Autodesk Inventor part; units mm, degrees
ref_plane "YZ Plane" through (0, 0, 0) normal (1, 0, 0) x (0, 1, 0)
ref_plane "XZ Plane" through (0, 0, 0) normal (0, 1, 0) x (-1, 0, 0)
ref_plane "XY Plane" through (0, 0, 0) normal (0, 0, 1) x (1, 0, 0)
sketch "Sketch1" plane through (0, 0, 0) normal (0, 0, 1) x (1, 0, 0)
  circle A0 centre (0, 0) radius 11.1125
  line L0 (0, 0) -> (7.6256, 0)
  line L1 (-3.8526, 6.604) -> (3.8128, 6.604)
  line L2 (3.8128, 6.604) -> (7.6256, 0)
  line L3 (7.6256, 0) -> (3.8128, -6.604)
  line L4 (3.8128, -6.604) -> (-3.8128, -6.604)
  line L5 (-3.8128, -6.604) -> (-7.6056, -0.0348)
  line L6 (-7.6056, -0.0348) -> (-3.8526, 6.604)
  line L7 (0, 0) -> (0, 6.604)
  line L8 (0, 0) -> (0, -6.604)
  line L9 (0, 0) -> (-5.7192, 3.302)
  line L10 (0, 0) -> (5.7192, -3.302)
  line L11 (0, 0) -> (5.7192, 3.302)
  line L12 (0, 0) -> (-5.7192, -3.302)
  line L13 (-7.2737, 0.1016) -> (-3.7248, 6.2484)
  line L14 (-3.5489, 6.35) -> (3.5489, 6.35)
  arc A1 (3.7248, 6.2484) -> (3.5489, 6.35) centre (3.5489, 6.1468) ccw
  line L15 (3.7248, 6.2484) -> (7.2737, 0.1016)
  arc A2 (-3.5489, 6.35) -> (-3.7248, 6.2484) centre (-3.5489, 6.1468) ccw
  arc A3 (-7.2737, 0.1016) -> (-7.2737, -0.1016) centre (-7.0977, 0) ccw
  line L16 (-3.7248, -6.2484) -> (-7.2737, -0.1016)
  line L17 (3.5489, -6.35) -> (-3.5489, -6.35)
  arc A4 (-3.7248, -6.2484) -> (-3.5489, -6.35) centre (-3.5489, -6.1468) ccw
  arc A5 (3.5489, -6.35) -> (3.7248, -6.2484) centre (3.5489, -6.1468) ccw
  line L18 (7.2737, -0.1016) -> (3.7248, -6.2484)
  arc A6 (7.2737, -0.1016) -> (7.2737, 0.1016) centre (7.0977, 0) ccw
  point P0 (0, 0)
  dimension "d0" = 22.225
  dimension "d19" = 6.604
  dimension "d20" = 6.604
  dimension "d21" = 6.604
  dimension "d22" = 6.604
  dimension "d23" = 60
  dimension "d24" = 60
  dimension "d25" = 6.604
  dimension "d26" = 6.604
  dimension "d27" = 60
  dimension "d28" = 60
  dimension "d30" = 13.208
extrude "Extrusion1" add sketch "Sketch1" along normal blind 12.7
sketch "Sketch3" plane through (-3.8128, -6.604, 0) normal (0, 1, 0) x (1, 0, 0)
  line L0 (11.4385, -12.7) -> (7.6256, -12.7)
  line L1 (7.6256, 0) -> (0, 0)
  line L2 (7.6256, -12.7) -> (0, 0)
  line L3 (7.6256, 0) -> (7.6256, -12.7)
  line L4 (0, 0) -> (7.6256, 0)
  line L5 (7.6256, 0) -> (7.6256, -12.7)
  line L6 (7.6256, -12.7) -> (0, -12.7)
  line L7 (7.6256, -12.7) -> (0, -12.7)
  line L8 (0, -12.7) -> (7.6256, 0)
  line L9 (0, 0) -> (0, -12.7)
  circle A0 centre (3.8128, -6.35) radius 1.27
  point P0 (3.8128, 0)
  dimension "d31" = 2.54
extrude "Extrusion2" cut sketch "Sketch3" against normal through all contours A0 L2 L8 | L8 L2 A0 | L2 L8 A0 | A0 L8 L2
properties part number "Churro Spacer"
Part model, mm, in its own coordinate system. A direction names the side the tool comes from. Coordinates: 2 decimals unless noted, no trailing zeros. Loops run counter-clockwise (first coordinate to the right, second up) from the corner with the lowest first, then second, coordinate; pieces in that order, holes last. Notation, with made-up numbers: M 26,33 L 36,33 A5 cw 36,37 Z; hole C 27.25,-29.5 d4. An arc over 180 degrees is marked long. Use a Markdown table: item, result. Add a question column.
Q1. Mould opens along Y. For faces 4 (the flat face through (0, -6.604, 8)), 5 (the cylindrical face through (10.6, -3.34, 6.26)), 6 (the flat face through (-5, -5, 12.7)) say: +Y half, -Y half, draft (parallel to the pull), parting line (faces both ways), or undercut.
Q2. Pin check, flat tips, straight feed: P1, Ø3, axis at y = 5.5, z = 5.5, coming from the -X side; P2, Ø4, axis at x = 2, z = 9, coming from the -Y side; P3, Ø6, axis at x = -3.5, z = 5.5, coming from the +Y side; P4, Ø3, axis at x = 5.5, z = 6.5, coming from the +Y side. Stop position of each tip, or through.
Q3. Cut at B-B (x = 6.25). Write the cut outline in (y, z), and give its area (3 significant figures).
Q4. Cut at D-D (x = 0). Write the cut outline in (y, z), and give its area (3 significant figures).
Q5. Probe L1, parallel to Z at x = 0, y = -10; L2, parallel to X at y = -1.75, z = 4; L3, parallel to X at y = -9.55, z = 6.35. List the from-to ranges inside material, lowest first.
Q6. Which spindle directions (+Z, -Z, +X, -X, +Y, -Y) get a long thin tool onto all of the face, cutting with end or side? Do faces 1 (the cylindrical face through (-0.28, -8.83, 7.59)), 2 (the flat face through (-5, -5, 0)), 3 (the flat face through (5.746, -3.256, 6.261)). Say none if no direction does.
Q7. Cut at A-A (y = 4.75). Write the cut outline in (x, z), and give its area (3 significant figures).
Q8. Cut at C-C (z = 2.5). Write the cut outline in (x, y) (1 decimal), and give its area (3 significant figures).
Worked out:
| question | item | result |
|---|---|---|
| 1 | face 4 | undercut |
| 1 | face 5 | parting line |
| 1 | face 6 | draft |
| 2 | P1 | stops at x = -10.37 |
| 2 | P2 | stops at y = -11.11 |
| 2 | P3 | stops at y = 11.1 |
| 2 | P4 | stops at y = 10.37 |
| 3 | outline | M -9.19,0 L -2.38,0 L -2.38,12.7 L -9.19,12.7 Z; M 2.38,0 L 9.19,0 L 9.19,12.7 L 2.38,12.7 Z |
| 3 | area | 173 mm2 |
| 4 | outline | M -11.11,0 L -6.6,0 L -6.6,5.08 L -11.11,5.08 Z; M -11.11,7.62 L -6.6,7.62 L -6.6,12.7 L -11.11,12.7 Z; M 6.6,0 L 11.11,0 L 11.11,12.7 L 6.6,12.7 Z |
| 4 | area | 103 mm2 |
| 5 | L1 | z = 0 to 5.08, 7.62 to 12.7 |
| 5 | L2 | x = -10.97 to -6.62, 6.62 to 10.97 |
| 5 | L3 | x = -5.68 to -1.27, 1.27 to 5.68 |
| 6 | face 1 | -Y |
| 6 | face 2 | -Z, +X, -X, +Y, -Y |
| 6 | face 3 | +Z, -Z |
| 7 | outline | M -10.05,0 L -4.9,0 L -4.9,12.7 L -10.05,12.7 Z; M 4.88,0 L 10.05,0 L 10.05,12.7 L 4.88,12.7 Z |
| 7 | area | 131 mm2 |
| 8 | outline | C 0,0 d22.2; hole M -7.6,0 L -3.8,-6.6 L 3.8,-6.6 L 7.6,0 L 3.8,6.6 L -3.9,6.6 Z |
| 8 | area | 237 mm2 |
